```python
from build123d import *

# Parameters (mm, degrees)
F1_DEPTH = 127
F3_DEPTH = 127
F5_DEPTH = 381
F6_DEPTH = 254


with BuildPart() as f1:
    # F0 (on Top) → F1 (new body)
    with BuildSketch(Plane.XY):
        Polygon((508, 254), (0, 254), (0, -381), (317.5, -381), (317.5, -508), (508, -508), align=None)
    extrude(amount=F1_DEPTH)

    # F2 (on face) → F3 (join)
    with BuildSketch(Plane(origin=(0, 0, 0), x_dir=(0, -1, 0), z_dir=(-1, 0, 0))):
        Polygon((-254, 1016), (-254, 127), (381, 127), (127, 1016), align=None)
    extrude(amount=-F3_DEPTH)

    # F4 (on face) → F5 (join)
    with BuildSketch(Plane(origin=(0, 254, 0), x_dir=(-1, 0, 0), z_dir=(0, 1, 0))):
        Polygon((-508, 127), (-127, 127), (-127, 762), align=None)
    extrude(amount=-F5_DEPTH)

    # F4 (on face) → F6 (cut)
    with BuildSketch(Plane(origin=(0, 254, 0), x_dir=(-1, 0, 0), z_dir=(0, 1, 0))):
        Polygon((-508, 127), (-127, 127), (-127, 762), align=None)
    extrude(amount=-F6_DEPTH, mode=Mode.SUBTRACT)


solid = f1.part
```
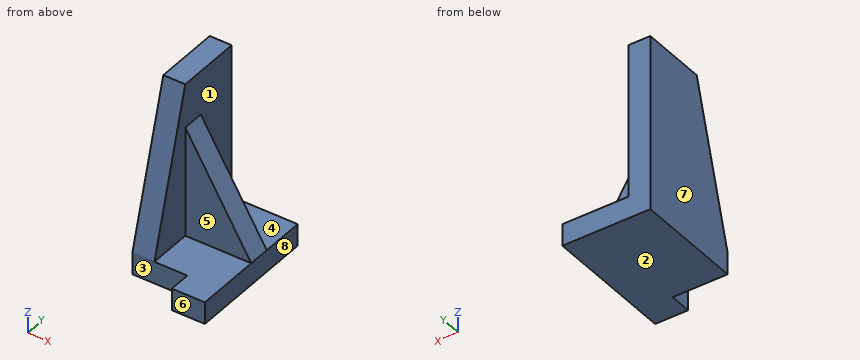
Here's how the part is built. I have some questions about the finished solid (model axes, mm). Face numbers are marked on the shaded views. A direction names the side the tool comes from. Coordinates: 2 decimals unless noted, no trailing zeros. Loops run counter-clockwise (first coordinate to the right, second up) from the corner with the lowest first, then second, coordinate; pieces in that order, holes last. Notation, with made-up numbers: (53.5, -21) - (102.5, -21) arc R9 cw to (102.5, -16) - close; hole circle Ø5 at (-15, -11.75). An arc over 180 degrees is marked (long way). Return JSON: item names as keys, results as strings. Group by question number.
Item 1: We'd pull the mould along X, two halves only. Please class the marked faces 6, 7 and 8: +X half, -X half, draft (parallel to the pull), parting line (faces both ways), or undercut.
Item 2: If we section it at D-D on y = -93: Write out the boundary of the cut face in (x, z).
Item 3: If we section it at B-B on y = -184: Write out the boundary of the cut face in (x, z), and give its area (3 significant figures).
Item 4: I need wall thicknesses on line 1 (X direction, y = 190.5, z = 902.5); line 2 (Y direction, x = 257, z = 473.5). Which ranges of each line are inside material? Lowest first, please. Write a range as from..to.
Item 5: If we section it at C-C on z = 513.5: Write out the boundary of the cut face in (x, y).
Item 6: On a 3-axis mill with a long thin cutter (end or side, diameter ignored), from which of +Z, -Z, +X, -X, +Y, -Y can I reach the whole of each face in a straight line? I mean the marked faces 1, 2, 3, 4 and 5. Say none if no direction works.
Item 7: Will these pins go through, and if not, where does the flat tip stop? P1, Ø12, axis at x = 283, y = -109.5, coming from the +Z side; P2, Ø10, axis at y = 53.5, z = 795, coming from the -X side; P3, Ø1, axis at x = 150.5, z = 359, coming from the -Y side; P4, Ø12, axis at y = 175, z = 437.5, coming from the +X side.
Item 8: If we section it at A-A on x = 181: Write out the boundary of the cut face in (y, z).
Calculated:
{
 "1": {"face 6": "draft", "face 7": "-X half", "face 8": "+X half"},
 "2": {"outline": "(0, 0) - (508, 0) - (508, 127) - (127, 762) - (127, 1016) - (0, 1016) - close"},
 "3": {"outline": "(0, 0) - (508, 0) - (508, 127) - (127, 127) - (127, 816.5) - (0, 816.5) - close", "area": "152,000 mm^2"},
 "4": {"line 1": "x = 0..127", "line 2": "y = -127..0"},
 "5": {"outline": "(0, -270.57) - (127, -270.57) - (127, -127) - (276.1, -127) - (276.1, 0) - (127, 0) - (127, 254) - (0, 254) - close"},
 "6": {"face 1": "+Z, +X", "face 2": "-Z, +X, -X, +Y, -Y", "face 3": "+Z, -Z, -X, -Y", "face 4": "+Z, +X, +Y", "face 5": "+Z, +X, -Y"},
 "7": {"P1": "stops at z = 512", "P2": "stops at x = 0", "P3": "stops at y = -127", "P4": "stops at x = 127"},
 "8": {"outline": "(-381, 0) - (254, 0) - (254, 127) - (0, 127) - (0, 672) - (-127, 672) - (-127, 127) - (-381, 127) - close"}
}
